```python
from build123d import *

# Parameters (mm, degrees)
ESQUISSE2_R                  = 10
ENL_V_MAT_EXTRU_1_DEPTH      = 687.62944883
R_P_TITION_CIRCULAIRE1_COUNT = 20
BOSS_EXTRU_1_START           = -10
ESQUISSE5_R                  = 436
ESQUISSE5_R_2                = 336
BOSS_EXTRU_1_DEPTH           = 10
BOSS_EXTRU_2_START           = 115
ESQUISSE6_R                  = 436
ESQUISSE6_R_2                = 426
BOSS_EXTRU_2_DEPTH           = 115
BOSS_EXTRU_3_START           = -10
BOSS_EXTRU_3_DEPTH           = 10
BOSS_EXTRU_4_START           = 115
BOSS_EXTRU_4_DEPTH           = 115
ENL_V_MAT_EXTRU_3_DEPTH      = 115
R_P_TITION_CIRCULAIRE6_COUNT = 2


with BuildPart() as part:
    # Esquisse1 → Révolution1 (revolve)
    with BuildSketch(Plane.XY, mode=Mode.PRIVATE) as r_volution1_sk:
        with BuildLine():
            Line((0, 0), (80, 0))
            Line((80, 0), (80, 52.5))
            ThreePointArc((80, 52.5), (70, 62.5), (80, 72.5))
            Line((80, 72.5), (80, 90))
            Line((80, 90), (0, 90))
            Line((0, 90), (0, 0))
        make_face()
    revolve(r_volution1_sk.sketch.rotate(Axis((-256, 27.419354839, 0), (0, -1, 0)), 90), axis=Axis((-256, 27.419354839, 0), (0, -1, 0)))

    # Esquisse2 → Enlèv. mat.-Extru.1 (cut, through all)
    with BuildSketch(Plane.XZ):
        with Locations(Location((40, 0, 0), (0, 0, 270))):
            Circle(ESQUISSE2_R)
    enl_v_mat_extru_1 = extrude(amount=-ENL_V_MAT_EXTRU_1_DEPTH, mode=Mode.SUBTRACT)

    # Répétition circulaire1: Enlèv. mat.-Extru.1 ×20 about axis
    r_p_tition_circulaire1_axis = Axis((-256, 0, 0), (0, 1, 0))
    for i in range(1, R_P_TITION_CIRCULAIRE1_COUNT):
        add(enl_v_mat_extru_1.rotate(r_p_tition_circulaire1_axis, i * 360 / R_P_TITION_CIRCULAIRE1_COUNT), mode=Mode.SUBTRACT)

    # Esquisse5 → Boss.-Extru.1 (add)
    with BuildSketch(Plane.XZ.offset(BOSS_EXTRU_1_START)):
        with Locations(Location((-256, 0, 0), (0, 0, 270))):
            Circle(ESQUISSE5_R)
        with Locations(Location((-256, 0, 0), (0, 0, 90))):
            Circle(ESQUISSE5_R_2, mode=Mode.SUBTRACT)
    extrude(amount=BOSS_EXTRU_1_DEPTH)

    # Esquisse6 → Boss.-Extru.2 (add)
    with BuildSketch(Plane(origin=(0, 10, 0), x_dir=(1, 0, 0), z_dir=(0, 1, 0)).offset(BOSS_EXTRU_2_START)):
        with Locations(Location((-256, 0, 0), (0, 0, 90))):
            Circle(ESQUISSE6_R)
        with Locations(Location((-256, 0, 0), (0, 0, 270))):
            Circle(ESQUISSE6_R_2, mode=Mode.SUBTRACT)
    extrude(amount=-BOSS_EXTRU_2_DEPTH)

    # Esquisse7 → Boss.-Extru.3 (add)
    with BuildSketch(Plane.XZ.offset(BOSS_EXTRU_3_START)):
        with BuildLine():
            Line((93.994285668, 260), (263.994285668, 260))
            Line((263.994285668, 260), (263.994285668, -260))
            Line((263.994285668, -260), (93.994285668, -260))
            ThreePointArc((93.994285668, -260), (180, 0), (93.994285668, 260))
        make_face()
    boss_extru_3 = extrude(amount=BOSS_EXTRU_3_DEPTH)

    # Esquisse8 → Boss.-Extru.4 (add)
    with BuildSketch(Plane(origin=(0, 10, 0), x_dir=(1, 0, 0), z_dir=(0, 1, 0)).offset(BOSS_EXTRU_4_START)):
        with BuildLine():
            Line((113.345366832, 250), (253.994285668, 250))
            Line((253.994285668, 250), (253.994285668, -250))
            Line((253.994285668, -250), (113.345366832, -250))
            Line((113.345366832, -250), (101.205823021, -250))
            ThreePointArc((101.205823021, -250), (97.635403251, -255.025491996), (93.994285668, -260))
            Line((93.994285668, -260), (263.994285668, -260))
            Line((263.994285668, -260), (263.994285668, 260))
            Line((263.994285668, 260), (93.994285668, 260))
            ThreePointArc((93.994285668, 260), (97.635403251, 255.025491996), (101.205823021, 250))
            Line((101.205823021, 250), (113.345366832, 250))
        make_face()
    boss_extru_4 = extrude(amount=-BOSS_EXTRU_4_DEPTH)

    # Esquisse9 → Enlèv. mat.-Extru.3 (cut)
    with BuildSketch(Plane(origin=(0, 125, 0), x_dir=(1, 0, 0), z_dir=(0, 1, 0))):
        with BuildLine():
            Line((101.205823021, -250), (88.928978197, -250))
            ThreePointArc((88.928978197, -250), (170, 0), (88.928978197, 250))
            Line((88.928978197, 250), (101.205823021, 250))
            ThreePointArc((101.205823021, 250), (180, 0), (101.205823021, -250))
        make_face()
    enl_v_mat_extru_3 = extrude(amount=-ENL_V_MAT_EXTRU_3_DEPTH, mode=Mode.SUBTRACT)

    # Répétition circulaire6: Boss.-Extru.3, Boss.-Extru.4, Enlèv. mat.-Extru.3 ×2 about axis
    r_p_tition_circulaire6_axis = Axis((-256, 0, 0), (0, 1, 0))
    add([boss_extru_3.rotate(r_p_tition_circulaire6_axis, i * 360 / R_P_TITION_CIRCULAIRE6_COUNT) for i in range(1, R_P_TITION_CIRCULAIRE6_COUNT)])
    add([boss_extru_4.rotate(r_p_tition_circulaire6_axis, i * 360 / R_P_TITION_CIRCULAIRE6_COUNT) for i in range(1, R_P_TITION_CIRCULAIRE6_COUNT)])
    add([enl_v_mat_extru_3.rotate(r_p_tition_circulaire6_axis, i * 360 / R_P_TITION_CIRCULAIRE6_COUNT) for i in range(1, R_P_TITION_CIRCULAIRE6_COUNT)], mode=Mode.SUBTRACT)


solid = part.part
```
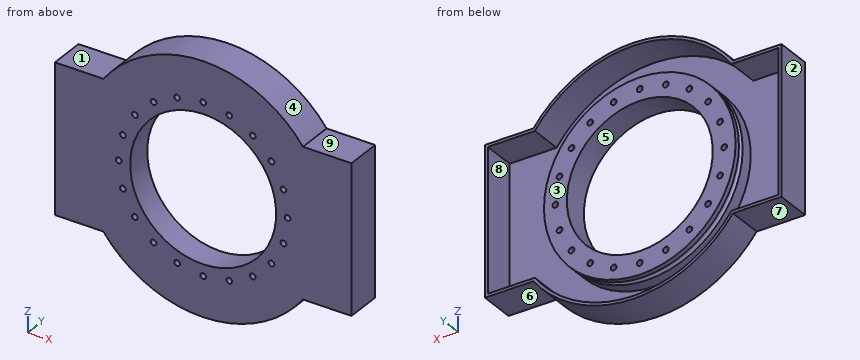
Could you check a few things on this model? Use its own coordinates, in mm. Face numbers are marked on the shaded views. A direction names the side the tool comes from. Round coordinates to 2 decimals unless told otherwise and drop trailing zeros. Write each loop counter-clockwise with the first axis right and the second up, starting at its lowest first coordinate (ties: lowest second). Pieces come first, ordered by that corner, then holes. Notation, with made-up numbers: M -5.75,60 L 6.25,60 A18 ccw 6.25,84 Z; hole C 31,57.25 d6. An arc over 180 degrees is marked long. Write each question's results on one line, items separated by ' | '. Start each with the question number.
1. I'm going to push flat-ended pins straight in: pin 1 Ø12 at (x, z) = (-429.98, 239.47) entering from +Y; pin 2 Ø12 at (x, z) = (-164.5, 291.5) entering from +Y; pin 3 Ø3 at (x, y) = (-515, 38) entering from -Z; pin 4 Ø1 at (x, y) = (149, 44.5) entering from +Z. Where does each tip first touch, or does it pass through?
2. I need wall thicknesses on L1, parallel to Z at x = -698.5, y = 64; L2, parallel to X at y = 24, z = 0; L3, parallel to Z at x = -112, y = 46. Which ranges of each line are inside material? Lowest first, please. Write a range as from..to.
3. Imagine slicing it at C-C on y = 34. Count the separate pieces of the cut face and the enclosed holes in it, and give its area (3 significant figures).
4. Imagine slicing it at A-A on y = 108. List the corners of the cut face in (x, z) for me, and give its area (3 significant figures).
5. Thinking about a two-plate mould opening in X: for the marked faces 1, 2, 3 and 4, which applies, +X half, -X half, draft (parallel to the pull), parting line (faces both ways), or undercut?
6. Imagine slicing it at D-D on z = 374. List the corners of the cut face in (x, y) for me, and give its area (3 significant figures).
7. Imagine slicing it at B-B on x = 149.5. List the corners of the cut face in (y, z) for me, and give its area (3 significant figures).
8. On a 3-axis mill with a long thin cutter (end or side, diameter ignored), from which of +Z, -Z, +X, -X, +Y, -Y can I reach the whole of each face in a straight line? I mean the marked faces 5, 6, 7, 8 and 9. Say none if no direction works.
Result sheet:
1) pin 1: passes through | pin 2: stops at y = 90 | pin 3: stops at z = -351.84 | pin 4: stops at z = 260
2) L1: z = -260..-250, 250..260 | L2: x = -775.99..-765.99, -592..-562, -542..-512, 0..30, 50..80, 253.99..263.99 | L3: z = -411.53..-400.92, -303.58..-211.66, 211.66..303.58, 400.92..411.53
3) separate pieces: 2 | enclosed holes: 22 | area: 176,000 mm^2
4) outline: M -775.99,-260 L -605.99,-260 A436 ccw 93.99,-260 L 263.99,-260 L 263.99,260 L 93.99,260 A436 ccw -605.99,260 L -775.99,260 Z; hole M -765.99,-250 L -600.93,-250 A426 ccw 88.93,-250 L 253.99,-250 L 253.99,250 L 88.93,250 A426 ccw -600.93,250 L -765.99,250 Z | area: 33,100 mm^2
5) face 1: draft | face 2: -X half | face 3: undercut | face 4: parting line
6) outline: M -480.1,0 L -31.9,0 L -31.9,125 L -52.04,125 L -52.04,10 L -459.96,10 L -459.96,125 L -480.1,125 Z | area: 9,110 mm^2
7) outline: M 0,-260 L 125,-260 L 125,-250 L 10,-250 L 10,250 L 125,250 L 125,260 L 0,260 Z | area: 7,500 mm^2
8) face 5: +Y, -Y | face 6: -Z, +X, +Y, -Y | face 7: -Z, -X, +Y, -Y | face 8: +Y | face 9: +Z, +X, +Y, -Y
